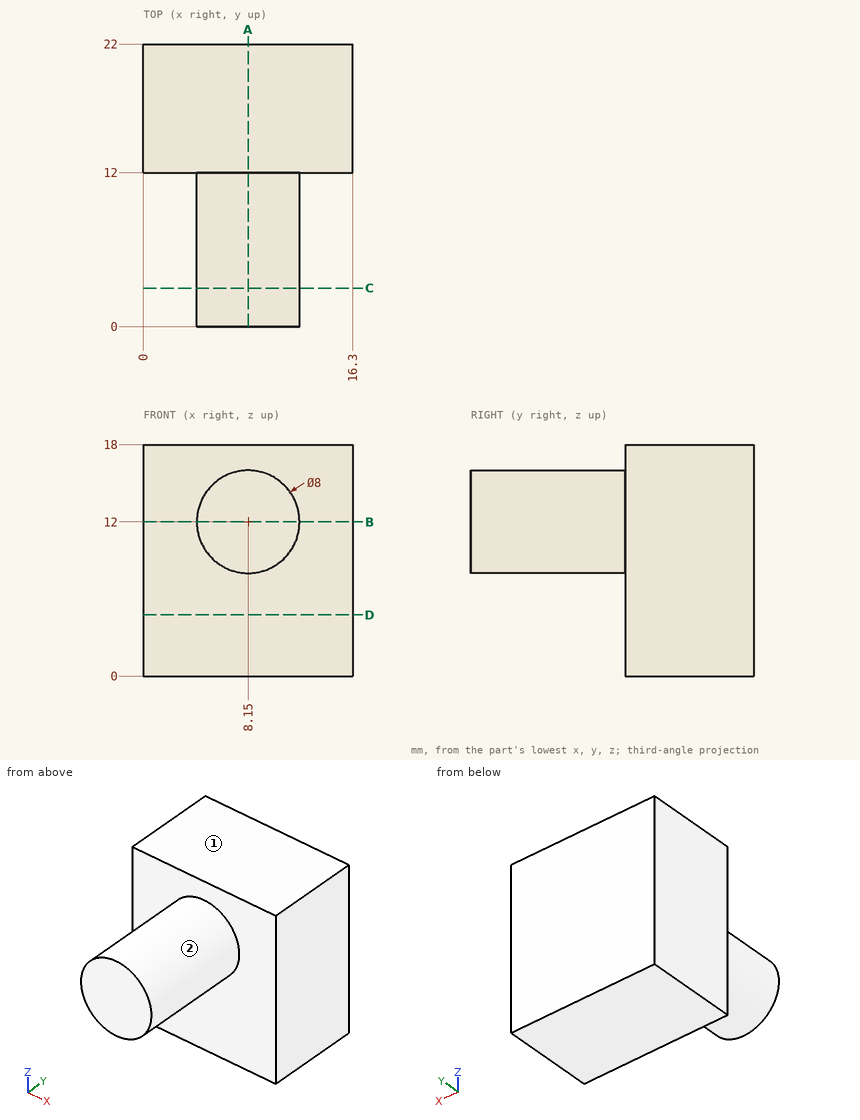
Part print with two shaded views. Sizes in mm from the minimum x, y, z corner. A direction names the side the tool comes from. Give positions to 0.01 mm unless a question says otherwise; leave off trailing zeros. Order: outer loops, then holes, each group sorted by start corner. A loop starts at its lowest first (then second) coordinate and runs counter-clockwise, first axis right, second up.
1) Saw through at A-A, the plane x = 8.15. Write the cut outline in (y, z), then the cut area to 3 significant figures.
2) 3-axis set-ups, long thin cutter, end or side, ignore diameter. For the marked faces 1 and 2: which of +Z, -Z, +X, -X, +Y, -Y reach the whole face in a straight line?
3) Pin check, flat tips, straight feed: pin 1 (8 mm diameter, centred on y = 5.5, z = 6.5, fed in from +X); pin 2 (4 mm diameter, centred on y = 14, z = 7.5, fed in from -X); pin 3 (5 mm diameter, centred on y = 2.5, z = 13, fed in from -X). Stop position of each tip, or through.
4) Saw through at D-D, the plane z = 4.75. Write the cut outline in (x, y).
5) Saw through at B-B, the plane z = 12. Write the cut outline in (x, y), then the cut area to 3 significant figures.
6) Wall check: probe 1 along Y at (x, z) = (3, 11); probe 2 along X at (y, z) = (10, 11.75); probe 3 along X at (y, z) = (6.5, 9.5). Give the ranges that are in metal, low to high.
7) Saw through at C-C, the plane y = 3. Write the cut outline in (x, z).
Computed:
1. outline: (0, 8) - (12, 8) - (12, 0) - (22, 0) - (22, 18) - (12, 18) - (12, 16) - (0, 16) - close
1. area: 276 mm2
2. face 1: +Z, +X, -X, +Y, -Y
2. face 2: -Y
3. pin 1: stops at x = 11.86
3. pin 2: stops at x = 0
3. pin 3: stops at x = 4.15
4. outline: (0, 12) - (16.3, 12) - (16.3, 22) - (0, 22) - close
5. outline: (0, 12) - (4.15, 12) - (4.15, 0) - (12.15, 0) - (12.15, 12) - (16.3, 12) - (16.3, 22) - (0, 22) - close
5. area: 259 mm2
6. probe 1: y = 12 to 22
6. probe 2: x = 4.16 to 12.14
6. probe 3: x = 5.03 to 11.27
7. outline: circle Ø8 at (8.15, 12)
